Here's the drawing with two shaded views (mm, measured from the low corner). I have some questions. Give positions to 0.01 mm unless a question says otherwise; leave off trailing zeros. Loops run counter-clockwise (first coordinate to the right, second up) from the corner with the lowest first, then second, coordinate; pieces in that order, holes last. Notation, with made-up numbers: (76, 8) - (104, 8) arc R20 cw to (104, 32) - close; hole circle Ø6 at (34, 81.5). An arc over 180 degrees is marked (long way). Use a Markdown table: item, result. Add a question column.
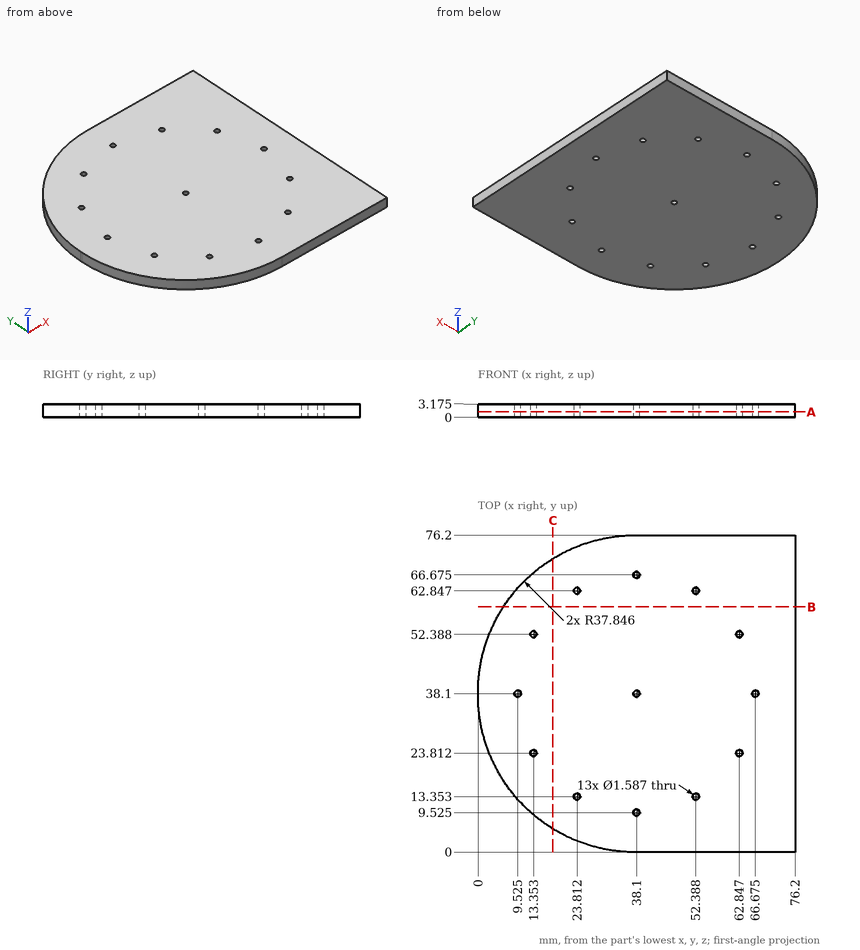
1. Will these pins go through, and if not, where does the flat tip stop? P1, Ø1.4, axis at x = 52.39, y = 13.35, coming from the +Z side; P2, Ø1.5, axis at x = 9.5, z = 2, coming from the -Y side (1 decimal).
2. Suppose I cut it at B-B (y = 59). List the corners of the cut face in (x, z) for me (1 decimal).
3. Please list where these lines run through material, in increasing order: line 1 along X through (y, z) = (38.1, 1.5); line 2 along Y through (x, z) = (13, 0.3) (1 decimal). Write a range as [from, to].
4. Suppose I cut it at A-A (z = 1.3). State how many separate pieces and enclosed holes the cut face has, and give its area (3 significant figures).
5. Suppose I cut it at C-C (x = 18). List the corners of the cut face in (y, z) for me (1 decimal).
Results below:
| question | item | result |
|---|---|---|
| 1 | P1 | through |
| 1 | P2 | y = 11.9 |
| 2 | outline | (6.1, 0) - (76.2, 0) - (76.2, 3.2) - (6.1, 3.2) - close |
| 3 | line 1 | [0, 8.73], [10.32, 37.31], [38.89, 65.88], [67.47, 76.2] |
| 3 | line 2 | [9.3, 23.1], [24.5, 51.7], [53.1, 66.9] |
| 4 | separate pieces | 1 |
| 4 | enclosed holes | 13 |
| 4 | area | 5,170 mm² |
| 5 | outline | (5.6, 0) - (70.6, 0) - (70.6, 3.2) - (5.6, 3.2) - close |
